```python
from build123d import *

# Parameters (mm, degrees)
CROQUIS2_R              = 17.5
SALIENTE_EXTRUIR1_DEPTH = 650
CROQUIS3_R              = 12.7
CORTAR_EXTRUIR1_DEPTH   = 640
REDONDEO1_R             = 3
CROQUIS4_W              = 0.7347375
CROQUIS4_H              = 0.188618068
SALIENTE_EXTRUIR2_DEPTH = 10


with BuildPart() as part:
    # Croquis2 → Saliente-Extruir1 (new body)
    with BuildSketch(Plane.XY):
        Circle(CROQUIS2_R)
    extrude(amount=-SALIENTE_EXTRUIR1_DEPTH)

    # Croquis3 → Cortar-Extruir1 (cut)
    with BuildSketch(Plane.XY):
        Circle(CROQUIS3_R)
    extrude(amount=-CORTAR_EXTRUIR1_DEPTH, mode=Mode.SUBTRACT)

    # Redondeo1
    redondeo1_edges = [part.edges().sort_by_distance(p)[0] for p in [
        (-17.5, 0, -650),
    ]]
    fillet(redondeo1_edges, radius=REDONDEO1_R)

    # Croquis4 → Saliente-Extruir2 (add)
    with BuildSketch(Plane.XY):
        with Locations((0, 17.5)):
            Rectangle(CROQUIS4_W, CROQUIS4_H)
    extrude(amount=-SALIENTE_EXTRUIR2_DEPTH)


solid = part.part
```
Geometry: final body of the model. Coordinates: model frame, mm. A direction names the side the tool comes from. Give positions to 0.01 mm unless a question says otherwise; leave off trailing zeros. Loops run counter-clockwise (first coordinate to the right, second up) from the corner with the lowest first, then second, coordinate; pieces in that order, holes last. Notation, with made-up numbers: (10.5, 21) -> (60.5, 21) arc R27 ccw to (60.5, 42) -> close; hole circle Ø8 at (30.25, -1). An arc over 180 degrees is marked (long way). Use one line per item in the form item = value.
Item 1: Section query A-A on y = 0. Output: boundary loops of the cut face in (x, z), and give its area (3 significant figures).
A:
outline = (-17.5, -647) arc R3 ccw to (-14.5, -650) -> (14.5, -650) arc R3 ccw to (17.5, -647) -> (17.5, 0) -> (12.7, 0) -> (12.7, -640) -> (-12.7, -640) -> (-12.7, 0) -> (-17.5, 0) -> close
area = 6,490 mm^2
Item 2: Line query: probe 1 along Y at (x, z) = (0, -277); probe 2 along Z at (x, y) = (8, 8.5); probe 3 along Z at (x, y) = (-14.5, -3). Output: solid intervals per line, ascending.
A:
probe_1 = -17.5 to -12.7, 12.7 to 17.5
probe_2 = -650 to -640
probe_3 = -649.98 to 0
Item 3: Access query for faces 1 (the face through (0, 0, -640)), 2 (the face through (0, 0, -650)). Directions: +Z, -Z, +X, -X, +Y, -Y. A direction counts if a zero-diameter tool reaches every point of the face in a straight line with its end or side. Return the directions, or none.
A:
face_1 = +Z
face_2 = -Z, +X, -X, +Y, -Y
Item 4: Section query B-B on z = -575. Output: boundary loops of the cut face in (x, y).
A:
outline = circle Ø35 at (0, 0); hole circle Ø25.4 at (0, 0)
Item 5: Pin query (flat end, axial travel): P1, Ø3, axis at y = -9.5, z = -560.5, coming from the -X side; P2, Ø3, axis at x = -7, z = -479, coming from the +Y side; P3, Ø3, axis at y = 10, z = -134.5, coming from the -X side; P4, Ø20.5, axis at x = 3.5, y = 4.5, coming from the +Z side. Return the tip coordinate at first contact, or that it passes through.
A:
P1 = -15.56
P2 = 16.61
P3 = -15.3
P4 = 0
